Can you work these out from the model? Positions are in its coordinate system, mm. Face numbers are marked on the shaded views. A direction names the side the tool comes from. Coordinates: 2 decimals unless noted, no trailing zeros. Loops run counter-clockwise (first coordinate to the right, second up) from the corner with the lowest first, then second, coordinate; pieces in that order, holes last. Notation, with made-up numbers: (85, -31.5) -> (117, -31.5) arc R13 ccw to (117, -26.5) -> close; hole circle Ø10 at (-13.5, 63). An arc over 180 degrees is marked (long way). Put each result on its own line as item: value. Start each with the question number.
Item 1: If we section it at D-D on y = 14: Please give me the cut outline in (x, z), plus the area to 3 significant figures.
Item 2: If we section it at A-A on y = 0: Please give me the cut outline in (x, z).
Item 3: Please list where these lines run through material, in increasing order: L1, parallel to Z at x = 6.5, y = -13.5; L2, parallel to X at y = 0.5, z = 68.5; L3, parallel to X at y = -3.5, z = 68.5. Write a range as from..to.
Item 4: If we section it at C-C on z = 9.5: Please give me the cut outline in (x, y), plus the area to 3 significant figures.
Item 5: If we section it at B-B on x = 0: Please give me the cut outline in (y, z).
Item 6: For the marked faces 1 and 2, which set-ups out of +Z, -Z, +X, -X, +Y, -Y let a thin tool reach every point of the face, with its end or its side?
Item 7: We'd pull the mould along Z, two halves only. Please class the marked faces 3, 4, 5 and 6: pulls with the +Z half, pulls with the -Z half, needs draft (parallel to the pull), parting line crosses it, or undercut.
Item 8: Will these pins go through, and if not, where does the flat tip stop? P1, Ø8, axis at y = 5, z = 42.5, coming from the -X side; P2, Ø3, axis at x = 1, z = 51.5, coming from the -Y side; P3, Ø1.8, axis at y = -1.5, z = 64, coming from the +X side.
```python
from build123d import *

# Parameters (mm, degrees)
F0_R          = 17.5
F1_DEPTH      = 5
F2_R          = 12.5
F3_DEPTH      = 72
F4_W          = 10
F4_H          = 6
F5_DEPTH      = 17.501
F5_DEPTH_BACK = 17.501
F6_SIZE2      = 2
F6_SIZE       = 2


with BuildPart() as f1:
    # F0 (on Top) → F1 (new body)
    with BuildSketch(Plane.XY):
        Circle(F0_R)
    extrude(amount=F1_DEPTH)

    # F2 (on Top) → F3 (join)
    with BuildSketch(Plane.XY):
        Circle(F2_R)
    extrude(amount=F3_DEPTH)

    # F4 (on Front) → F5 (cut, two sides)
    with BuildSketch(Plane.XZ) as f5_sk:
        with Locations((11.5, 63)):
            Rectangle(F4_W, F4_H)
    extrude(amount=-F5_DEPTH, mode=Mode.SUBTRACT)
    extrude(f5_sk.sketch, amount=F5_DEPTH_BACK, mode=Mode.SUBTRACT)

    # F6
    f6_edges = [f1.edges().sort_by_distance(p)[0] for p in [
        (-12.5, 0, 72),
    ]]
    chamfer(f6_edges, length=F6_SIZE, length2=F6_SIZE2)


solid = f1.part
```
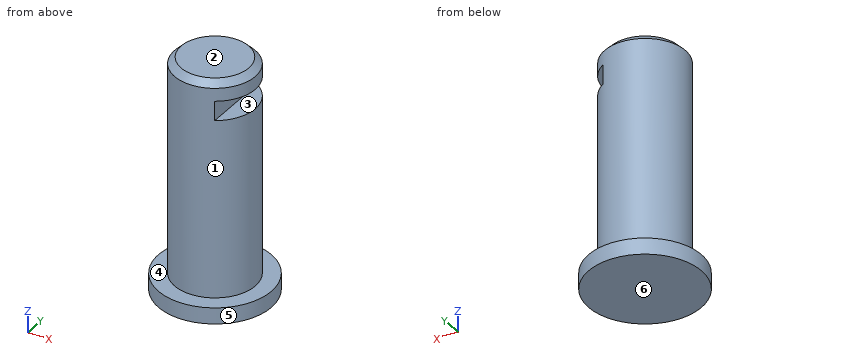
Solutions:
1. outline: (-10.5, 0) -> (10.5, 0) -> (10.5, 5) -> (-10.5, 5) -> close
1. area: 105 mm^2
2. outline: (-17.5, 0) -> (17.5, 0) -> (17.5, 5) -> (12.5, 5) -> (12.5, 60) -> (6.5, 60) -> (6.5, 66) -> (12.5, 66) -> (12.5, 70) -> (10.5, 72) -> (-10.5, 72) -> (-12.5, 70) -> (-12.5, 5) -> (-17.5, 5) -> close
3. L1: 0..5
3. L2: -12.49..12.49
3. L3: -12..12
4. outline: circle Ø25 at (0, 0)
4. area: 491 mm^2
5. outline: (-17.5, 0) -> (17.5, 0) -> (17.5, 5) -> (12.5, 5) -> (12.5, 70) -> (10.5, 72) -> (-10.5, 72) -> (-12.5, 70) -> (-12.5, 5) -> (-17.5, 5) -> close
6. face 1: +Z
6. face 2: +Z, +X, -X, +Y, -Y
7. face 3: undercut
7. face 4: pulls with the +Z half
7. face 5: needs draft
7. face 6: pulls with the -Z half
8. P1: x = -12.46
8. P2: y = -12.5
8. P3: x = 6.5
